Part model, mm, in its own coordinate system. A direction names the side the tool comes from. Give positions to 0.01 mm unless a question says otherwise; leave off trailing zeros. Write each loop counter-clockwise with the first axis right and the second up, starting at its lowest first coordinate (ties: lowest second). Pieces come first, ordered by that corner, then holes. Notation, with made-up numbers: M -29.5,1.25 L 19.5,1.25 A26 cw 19.5,36.25 Z; hole C 5.5,30.5 d8. An arc over 180 degrees is marked long. Use a Markdown table: item, result. Add a question column.
from build123d import *
from OCP.BRepFilletAPI import BRepFilletAPI_MakeChamfer

# Parameters (mm, degrees)
DODANIE_WYCI_GNI_CIE1_DEPTH      = 23.5
DODANIE_WYCI_GNI_CIE1_DEPTH_BACK = 23.5
SZKIC1_W                         = 33
SZKIC1_H                         = 15
SZKIC2_W                         = 35
SZKIC2_H                         = 15
WYTNIJ_WYCI_GNI_CIE1_DEPTH       = 42.200728149
SZKIC3_R                         = 1.75
WYTNIJ_WYCI_GNI_CIE2_DEPTH       = 51.373604199
SZKIC4_W                         = 33
SZKIC4_H                         = 47
DODANIE_WYCI_GNI_CIE2_DEPTH      = 8
SZKIC5_R                         = 6.2
SZKIC5_W                         = 11
SZKIC5_H                         = 21
WYTNIJ_WYCI_GNI_CIE3_DEPTH       = 9
DODANIE_WYCI_GNI_CIE3_DEPTH      = 8
SZKIC8_R                         = 1.25
WYTNIJ_WYCI_GNI_CIE4_DEPTH       = 9
SZKIC10_R                        = 2.2
WYTNIJ_WYCI_GNI_CIE5_DEPTH       = 2
SZKIC11_R                        = 1.75
DODANIE_WYCI_GNI_CIE4_DEPTH      = 10
SZKIC12_R                        = 1.85
WYTNIJ_WYCI_GNI_CIE6_DEPTH       = 58.725644215
WYTNIJ_WYCI_GNI_CIE7_DEPTH       = 6
SFAZOWANIE1_SIZE                 = 24.5
SFAZOWANIE1_SIZE_2               = 15
ZAOKR_GLENIE1_R                  = 10
SFAZOWANIE2_SIZE                 = 4
SZKIC14_R                        = 4.5
WYTNIJ_WYCI_GNI_CIE8_DEPTH       = 1.5


# Some blends are built 0.0001 mm under size
with BuildPart() as part:
    # Szkic1 → Dodanie-wyci_gni_cie1 (new, two sides: drawn at the far end of the back side and taken through both)
    with BuildSketch(Plane.XY.offset(-DODANIE_WYCI_GNI_CIE1_DEPTH_BACK)):
        Rectangle(SZKIC1_W, SZKIC1_H)
    extrude(amount=DODANIE_WYCI_GNI_CIE1_DEPTH + DODANIE_WYCI_GNI_CIE1_DEPTH_BACK)

    # Szkic2 → Wytnij-wyci_gni_cie1 (cut, through all)
    with BuildSketch(Plane(origin=(16.5, 0, 0), x_dir=(0, 0, -1), z_dir=(1, 0, 0))):
        Rectangle(SZKIC2_W, SZKIC2_H)
    extrude(amount=-WYTNIJ_WYCI_GNI_CIE1_DEPTH, mode=Mode.SUBTRACT)


with BuildPart() as wytnij_wyci_gni_cie1_piece_1:
    # of the separate pieces the step leaves, piece 1, a body of its own (wytnij_wyci_gni_cie1_pieces)
    add(part.part.solids().sort_by_distance((-16.5, -7.5, -17.5))[0])


with BuildPart() as wytnij_wyci_gni_cie1_piece_2:
    # of the separate pieces the step leaves, piece 2, a body of its own (wytnij_wyci_gni_cie1_pieces)
    add(part.part.solids().sort_by_distance((-16.5, -7.5, 23.5))[0])


with BuildPart() as wytnij_wyci_gni_cie2_tool:
    # Szkic3 → Wytnij-wyci_gni_cie2 (new, through all)
    with BuildSketch(Plane.XY.offset(23.5)):
        with Locations((-4.3, -2.5)):
            Circle(SZKIC3_R)
        with Locations((4.3, -2.5)):
            Circle(SZKIC3_R)
    extrude(amount=-WYTNIJ_WYCI_GNI_CIE2_DEPTH)


with BuildPart() as wytnij_wyci_gni_cie1_piece_1_1:
    add(wytnij_wyci_gni_cie1_piece_1.part)

    # Wytnij-wyci_gni_cie2: cut by wytnij_wyci_gni_cie2_tool
    add(wytnij_wyci_gni_cie2_tool.part, mode=Mode.SUBTRACT)



with BuildPart() as wytnij_wyci_gni_cie1_piece_2_1:
    add(wytnij_wyci_gni_cie1_piece_2.part)

    # Wytnij-wyci_gni_cie2: cut by wytnij_wyci_gni_cie2_tool
    add(wytnij_wyci_gni_cie2_tool.part, mode=Mode.SUBTRACT)


with BuildPart() as wytnij_wyci_gni_cie1_piece_1_2:
    add(wytnij_wyci_gni_cie1_piece_1_1.part)

    add(wytnij_wyci_gni_cie1_piece_2_1.part)  # Dodanie-wyci_gni_cie2 merges Wytnij-wyci_gni_cie1 piece 2
    # Szkic4 → Dodanie-wyci_gni_cie2 (add)
    with BuildSketch(Plane(origin=(0, 7.5, 0), x_dir=(1, 0, 0), z_dir=(0, 1, 0))):
        Rectangle(SZKIC4_W, SZKIC4_H)
    extrude(amount=DODANIE_WYCI_GNI_CIE2_DEPTH)

    # Szkic5 → Wytnij-wyci_gni_cie3 (cut)
    with BuildSketch(Plane(origin=(0, 15.5, 0), x_dir=(1, 0, 0), z_dir=(0, 1, 0))):
        with Locations(Location((0, 0, 0), (0, 0, 270))):
            Circle(SZKIC5_R)
        with Locations((-16.5, 0)):
            Rectangle(SZKIC5_W, SZKIC5_H)
    extrude(amount=-WYTNIJ_WYCI_GNI_CIE3_DEPTH, mode=Mode.SUBTRACT)

    # Szkic7 → Dodanie-wyci_gni_cie3 (add)
    with BuildSketch(Plane(origin=(0, 15.5, 0), x_dir=(1, 0, 0), z_dir=(0, 1, 0))):
        Polygon((-16.5, 10.5), (-16.5, 23.5), (-33, 23.5), (-41, 23.5), (-41, -23.5), (-33, -23.5), (-16.5, -23.5), (-16.5, -10.5), (-33, -10.5), (-33, 10.5), align=None)
    extrude(amount=-DODANIE_WYCI_GNI_CIE3_DEPTH)

    # Szkic8 → Wytnij-wyci_gni_cie4 (cut)
    with BuildSketch(Plane(origin=(0, 15.5, 0), x_dir=(1, 0, 0), z_dir=(0, 1, 0))):
        with Locations(Location((-30.5, -13.5, 0), (0, 0, 270))):
            Circle(SZKIC8_R)
        with Locations(Location((-36, -8, 0), (0, 0, 270))):
            Circle(SZKIC8_R)
        with Locations(Location((-22.5, -13.5, 0), (0, 0, 270))):
            Circle(SZKIC8_R)
        with Locations(Location((-14.5, -13.5, 0), (0, 0, 270))):
            Circle(SZKIC8_R)
        with Locations(Location((-6.5, -13.5, 0), (0, 0, 270))):
            Circle(SZKIC8_R)
    wytnij_wyci_gni_cie4 = extrude(amount=-WYTNIJ_WYCI_GNI_CIE4_DEPTH, mode=Mode.SUBTRACT)

    # Szkic10 → Wytnij-wyci_gni_cie5 (cut)
    with BuildSketch(Plane.XZ.offset(-7.5)):
        with Locations(Location((-36, 8, 0), (0, 0, 270))):
            Circle(SZKIC10_R)
        with Locations(Location((-30.5, 13.5, 0), (0, 0, 270))):
            Circle(SZKIC10_R)
        with Locations(Location((-22.5, 13.5, 0), (0, 0, 270))):
            Circle(SZKIC10_R)
        with Locations(Location((-14.5, 13.5, 0), (0, 0, 270))):
            Circle(SZKIC10_R)
        with Locations(Location((-6.5, 13.5, 0), (0, 0, 270))):
            Circle(SZKIC10_R)
    wytnij_wyci_gni_cie5 = extrude(amount=-WYTNIJ_WYCI_GNI_CIE5_DEPTH, mode=Mode.SUBTRACT)

    # Lustro2: Wytnij-wyci_gni_cie4, Wytnij-wyci_gni_cie5 across plane
    add(wytnij_wyci_gni_cie4.mirror(Plane.XY), mode=Mode.SUBTRACT)
    add(wytnij_wyci_gni_cie5.mirror(Plane.XY), mode=Mode.SUBTRACT)

    # Szkic11 → Dodanie-wyci_gni_cie4 (add)
    with BuildSketch(Plane.XY.offset(23.5)):
        Polygon((-16.5, 7.5), (-16.5, -7.5), (16.5, -7.5), (16.5, 15.5), (-41, 15.5), (-41, 7.5), align=None)
        with Locations((-4.3, -2.5)):
            Circle(SZKIC11_R, mode=Mode.SUBTRACT)
        with Locations((4.3, -2.5)):
            Circle(SZKIC11_R, mode=Mode.SUBTRACT)
    dodanie_wyci_gni_cie4 = extrude(amount=DODANIE_WYCI_GNI_CIE4_DEPTH)

    # Szkic12 → Wytnij-wyci_gni_cie6 (cut, through all)
    with BuildSketch(Plane.XZ.offset(7.5)):
        with Locations(Location((-12.5, 25.5, 0), (0, 0, 270))):
            Circle(SZKIC12_R)
        with Locations(Location((10.5, 25.5, 0), (0, 0, 270))):
            Circle(SZKIC12_R)
    wytnij_wyci_gni_cie6 = extrude(amount=-WYTNIJ_WYCI_GNI_CIE6_DEPTH, mode=Mode.SUBTRACT)

    # Szkic13 → Wytnij-wyci_gni_cie7 (cut)
    with BuildSketch(Plane(origin=(0, 15.5, 0), x_dir=(1, 0, 0), z_dir=(0, 1, 0))):
        Polygon((-12.5, -22.035898385), (-15.5, -23.767949192), (-15.5, -27.232050808), (-12.5, -28.964101615), (-9.5, -27.232050808), (-9.5, -23.767949192), align=None)
        Polygon((10.5, -22.035898385), (7.5, -23.767949192), (7.5, -27.232050808), (10.5, -28.964101615), (13.5, -27.232050808), (13.5, -23.767949192), align=None)
    wytnij_wyci_gni_cie7 = extrude(amount=-WYTNIJ_WYCI_GNI_CIE7_DEPTH, mode=Mode.SUBTRACT)

    # Lustro6: Dodanie-wyci_gni_cie4, Wytnij-wyci_gni_cie6, Wytnij-wyci_gni_cie7 across plane
    add(dodanie_wyci_gni_cie4.mirror(Plane.XY))
    add(wytnij_wyci_gni_cie6.mirror(Plane.XY), mode=Mode.SUBTRACT)
    add(wytnij_wyci_gni_cie7.mirror(Plane.XY), mode=Mode.SUBTRACT)

    # Sfazowanie1
    sfazowanie1_edges_1 = [wytnij_wyci_gni_cie1_piece_1_2.edges().sort_by_distance(p)[0] for p in [
        (-16.5, 7.5, -28.5),
    ]]
    sfazowanie1_side_1 = [wytnij_wyci_gni_cie1_piece_1_2.faces().sort_by_distance(p)[0] for p in [
        (-16.8, 7.5, -28.5),
    ]]
    sfazowanie1_edges_2 = [wytnij_wyci_gni_cie1_piece_1_2.edges().sort_by_distance(p)[0] for p in [
        (-16.5, 7.5, 25.5),
    ]]
    sfazowanie1_side_2 = [wytnij_wyci_gni_cie1_piece_1_2.faces().sort_by_distance(p)[0] for p in [
        (-16.5, 7.2, 25.5),
    ]]
    sfazowanie1 = BRepFilletAPI_MakeChamfer(wytnij_wyci_gni_cie1_piece_1_2.part.solid().wrapped)
    for e in sfazowanie1_edges_1:
        sfazowanie1.Add(SFAZOWANIE1_SIZE - 0.0001, SFAZOWANIE1_SIZE_2 - 0.0001, e.wrapped, sfazowanie1_side_1[0].wrapped)
    for e in sfazowanie1_edges_2:
        sfazowanie1.Add(SFAZOWANIE1_SIZE_2 - 0.0001, SFAZOWANIE1_SIZE - 0.0001, e.wrapped, sfazowanie1_side_2[0].wrapped)
    add(Compound.cast(sfazowanie1.Shape()), mode=Mode.REPLACE)  # a hair under: the kernel refuses the full size

    # Zaokr_glenie1
    zaokr_glenie1_edges = [wytnij_wyci_gni_cie1_piece_1_2.edges().sort_by_distance(p)[0] for p in [
        (-41, 11.5, 33.5),
        (-41, 11.5, -33.5),
    ]]
    fillet(zaokr_glenie1_edges, radius=ZAOKR_GLENIE1_R)

    # Sfazowanie2
    # the kernel refuses this chamfer: 4 mm, written as the material it adds along each edge
    with BuildSketch(Plane(origin=(-51.286631952, 7.5, -17.5), x_dir=(0, 0.02749587661058627, 0.9996219169112968), z_dir=(1, 0, 0))) as sfazowanie2_piece_1_section:
        Polygon((SFAZOWANIE2_SIZE * 0.999621916911, SFAZOWANIE2_SIZE * 0.0274958766106), (-SFAZOWANIE2_SIZE * 0.0274958766106, SFAZOWANIE2_SIZE * 0.999621916911), (0, 0), align=None)
    sfazowanie2_piece_1 = extrude(amount=67.786631952, mode=Mode.PRIVATE)
    sfazowanie2_piece_1 = split(sfazowanie2_piece_1, bisect_by=Plane(origin=(-41, 6.15842539, -16.26773288), z_dir=(1, 0, 0)), keep=Keep.TOP, mode=Mode.PRIVATE)
    sfazowanie2_piece_1 = split(sfazowanie2_piece_1, bisect_by=Plane(origin=(-18.343955111, -6.370950809, -16.26773288), z_dir=(0.5221528778597931, 0.852851905164511, 0)), keep=Keep.TOP, mode=Mode.PRIVATE)
    sfazowanie2_piece_1 = sfazowanie2_piece_1 - Plane(origin=(-30.5, 6.15842539, -13.5), x_dir=(0, 0, 1), z_dir=(0, -1, 0)) * Cylinder(2.2, 152, mode=Mode.PRIVATE)
    sfazowanie2_piece_1 = sfazowanie2_piece_1 - Plane(origin=(-22.5, 6.15842539, -13.5), x_dir=(0, 0, 1), z_dir=(0, -1, 0)) * Cylinder(2.2, 152, mode=Mode.PRIVATE)
    sfazowanie2_piece_1 = sfazowanie2_piece_1 - Plane(origin=(-14.5, 6.15842539, -13.5), x_dir=(0, 0, 1), z_dir=(0, -1, 0)) * Cylinder(2.2, 152, mode=Mode.PRIVATE)
    sfazowanie2_piece_1 = sfazowanie2_piece_1 - Plane(origin=(-6.5, 6.15842539, -13.5), x_dir=(0, 0, 1), z_dir=(0, -1, 0)) * Cylinder(2.2, 152, mode=Mode.PRIVATE)
    add(sfazowanie2_piece_1)
    with BuildSketch(Plane(origin=(-51.286631952, 7.5, 17.5), x_dir=(0, 0.02749587661058627, -0.9996219169112968), z_dir=(1, 0, 0))) as sfazowanie2_piece_2_section:
        Polygon((SFAZOWANIE2_SIZE * 0.999621916911, -SFAZOWANIE2_SIZE * 0.0274958766106), (-SFAZOWANIE2_SIZE * 0.0274958766106, -SFAZOWANIE2_SIZE * 0.999621916911), (0, 0), align=None)
    sfazowanie2_piece_2 = extrude(amount=67.786631952, mode=Mode.PRIVATE)
    sfazowanie2_piece_2 = split(sfazowanie2_piece_2, bisect_by=Plane(origin=(-18.343955111, -6.370950809, 16.26773288), z_dir=(0.5221528778597931, 0.8528519051645109, 0)), keep=Keep.TOP, mode=Mode.PRIVATE)
    sfazowanie2_piece_2 = split(sfazowanie2_piece_2, bisect_by=Plane(origin=(-41, 6.15842539, 16.26773288), z_dir=(1, 0, 0)), keep=Keep.TOP, mode=Mode.PRIVATE)
    sfazowanie2_piece_2 = sfazowanie2_piece_2 - Plane(origin=(-30.5, 6.15842539, 13.5), x_dir=(0, 0, -1), z_dir=(0, -1, 0)) * Cylinder(2.2, 152, mode=Mode.PRIVATE)
    sfazowanie2_piece_2 = sfazowanie2_piece_2 - Plane(origin=(-22.5, 6.15842539, 13.5), x_dir=(0, 0, -1), z_dir=(0, -1, 0)) * Cylinder(2.2, 152, mode=Mode.PRIVATE)
    sfazowanie2_piece_2 = sfazowanie2_piece_2 - Plane(origin=(-14.5, 6.15842539, 13.5), x_dir=(0, 0, -1), z_dir=(0, -1, 0)) * Cylinder(2.2, 152, mode=Mode.PRIVATE)
    sfazowanie2_piece_2 = sfazowanie2_piece_2 - Plane(origin=(-6.5, 6.15842539, 13.5), x_dir=(0, 0, -1), z_dir=(0, -1, 0)) * Cylinder(2.2, 152, mode=Mode.PRIVATE)
    add(sfazowanie2_piece_2)

    # Szkic14 → Wytnij-wyci_gni_cie8 (cut)
    with BuildSketch(Plane.XZ.offset(7.5)):
        with Locations(Location((-12.5, 25.5, 0), (0, 0, 270))):
            Circle(SZKIC14_R)
        with Locations(Location((10.5, 25.5, 0), (0, 0, 270))):
            Circle(SZKIC14_R)
        with Locations(Location((10.5, -25.5, 0), (0, 0, 270))):
            Circle(SZKIC14_R)
        with Locations(Location((-12.5, -25.5, 0), (0, 0, 270))):
            Circle(SZKIC14_R)
    extrude(amount=-WYTNIJ_WYCI_GNI_CIE8_DEPTH, mode=Mode.SUBTRACT)


solid = wytnij_wyci_gni_cie1_piece_1_2.part
1. Tool access for faces 5 (the flat face through (-14, 12.5, 22.9)), 6 (the flat face through (-3, -1, -17.5)), 7 (the flat face through (-22, 12, 10.5)), 8 (the flat face through (8.6, -6, -26.4)): list every direction of +Z, -Z, +X, -X, +Y, -Y with a clear straight run to the whole face (end or side of a thin tool).
2. Cut at A-A (z = -25.5). Give the number of separate pieces and of enclosed holes in the cut face, then the cut area to 3 significant figures.
3. Cut at D-D (x = -36). Write the cut outline in (y, z).
4. Drill centre lines: probe 1 along X at (y, z) = (11.4, 8); probe 2 along X at (y, z) = (13.45, 13.5); probe 3 along Z at (x, y) = (-30.5, 7.4). Where is each one in solid material? Low to high. Write a range as [from, to].
5. Flat gauge pins, fed straight in: pin 1 (7 mm diameter, centred on x = 10.5, z = -25.5, fed in from -Y); pin 2 (1 mm diameter, centred on x = -3, z = 8.5, fed in from -Y); pin 3 (1.8 mm diameter, centred on x = 9, z = 25.5, fed in from +Y). Where does each tip first touch, or does it go through?
6. Mould opens along X. For faces 1 (the cylindrical face through (-23.72, 12.54, 13.23)), 2 (the flat face through (16.5, 10, 0)), 3 (the flat face through (-41, 12, 0)), 4 (the flat face through (-11, 9.5, -27)) say: released by +X, released by -X, zero draft, split by the parting line, or undercut.
A:
| question | item | result |
|---|---|---|
| 1 | face 5 | +Y |
| 1 | face 6 | +X, -X, -Y |
| 1 | face 7 | +Y, -Y |
| 1 | face 8 | -Y |
| 2 | separate pieces | 3 |
| 2 | enclosed holes | 2 |
| 2 | area | 904 mm² |
| 3 | outline | M 4.44,-32.16 L 15.5,-32.16 L 15.5,-9.25 L 9.5,-9.25 L 9.5,-10.2 L 7.5,-10.2 L 7.5,-13.5 L 4.44,-16.56 Z; M 4.44,16.56 L 7.5,13.5 L 7.5,10.2 L 9.5,10.2 L 9.5,9.25 L 15.5,9.25 L 15.5,32.16 L 4.44,32.16 Z; M 7.5,-5.8 L 9.5,-5.8 L 9.5,-6.75 L 15.5,-6.75 L 15.5,6.75 L 9.5,6.75 L 9.5,5.8 L 7.5,5.8 Z |
| 4 | probe 1 | x = [-41, -37.25], [-34.75, -33], [-11, 16.5] |
| 4 | probe 2 | x = [-41, -31.75], [-29.25, -23.75], [-21.25, -15.75], [-13.25, -7.75], [-5.25, 16.5] |
| 4 | probe 3 | z = [-33.5, -15.7], [15.7, 33.5] |
| 5 | pin 1 | stops at y = -6 |
| 5 | pin 2 | stops at y = 7.5 |
| 5 | pin 3 | stops at y = 9.5 |
| 6 | face 1 | undercut |
| 6 | face 2 | released by +X |
| 6 | face 3 | released by -X |
| 6 | face 4 | undercut |
